Part model, mm, in its own coordinate system. Face numbers are marked on the shaded views. A direction names the side the tool comes from. Coordinates: 2 decimals unless noted, no trailing zeros. Write each loop counter-clockwise with the first axis right and the second up, starting at its lowest first coordinate (ties: lowest second). Pieces come first, ordered by that corner, then holes. Notation, with made-up numbers: (0.5, -21.75) -> (19.5, -21.75) arc R30 ccw to (19.5, 15.25) -> close; hole circle Ø2 at (29.25, 28.5). An arc over 180 degrees is marked (long way). Write item = value, one per line.
from build123d import *

# Parameters (mm, degrees)
F0_R     = 3.75
F0_R_2   = 2.5
F1_DEPTH = 15
F2_DEPTH = 9
F4_DEPTH = 7


# Not quite as in the source:
# - a feature names something its author has since deleted; it is built from what else it names


with BuildPart() as f1:
    # F0 (on Top) → F1 (new body)
    with BuildSketch(Plane.XY):
        Circle(F0_R)
        Circle(F0_R_2, mode=Mode.SUBTRACT)
    extrude(amount=F1_DEPTH)

    # F0 (on Top) → F2 (join)
    with BuildSketch(Plane.XY):
        Polygon((4.1, -2.3671361037), (4.1, 2.3671361037), (0, 4.7342722074), (-4.1, 2.3671361037), (-4.1, -2.3671361037), (0, -4.7342722074), align=None)
        Circle(F0_R, mode=Mode.SUBTRACT)
        Circle(F0_R)
        Circle(F0_R_2, mode=Mode.SUBTRACT)
        Circle(F0_R_2)
    extrude(amount=-F2_DEPTH)

    # F3 (on face) → F4 (cut)
    with BuildSketch(Plane(origin=(0, 0, -9), x_dir=(1, 0, 0), z_dir=(0, 0, -1))):
        Polygon((-3.3, 2.829016319), (-3.3, 0), (-3.3, -2.829016319), (-2.484232335, -3.3), (0, -3.3), (2.484232335, -3.3), (3.3, -2.829016319), (3.3, 0), (3.3, 2.829016319), (2.484232335, 3.3), (0, 3.3), (-2.484232335, 3.3), align=None)
    extrude(amount=-F4_DEPTH, mode=Mode.SUBTRACT)


solid = f1.part
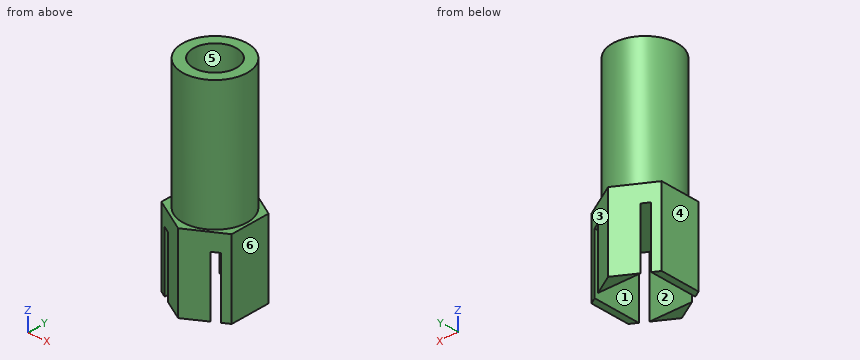
Q1. Which spindle directions (+Z, -Z, +X, -X, +Y, -Y) get a long thin tool onto all of the face, cutting with end or side? Do the marked faces 5 and 6. Say none if no direction does.
Model answer:
face_5 = +Z
face_6 = +Z, -Z, +X, +Y, -Y
Q2. Mould opens along X. For the marked faces 1, 2, 3 and 4 say: released by +X, released by -X, zero draft, split by the parting line, or undercut.
Model answer:
face_1 = undercut
face_2 = zero draft
face_3 = released by +X
face_4 = released by -X
Q3. Saw through at A-A on z = -6. Give the cut face in (x, y), and give its area (3 significant figures).
Model answer:
outline = (-4.1, -2.37) -> (-3.3, -2.83) -> (-3.3, 2.83) -> (-4.1, 2.37) -> close; (-2.48, -3.3) -> (0, -4.73) -> (2.48, -3.3) -> close; (-2.48, 3.3) -> (2.48, 3.3) -> (0, 4.73) -> close; (3.3, -2.83) -> (4.1, -2.37) -> (4.1, 2.37) -> (3.3, 2.83) -> close
area = 15.4 mm²
Q4. Saw through at D-D on z = -1. Give the cut face in (x, y), and give its area (3 significant figures).
Model answer:
outline = (-4.1, -2.37) -> (0, -4.73) -> (4.1, -2.37) -> (4.1, 2.37) -> (0, 4.73) -> (-4.1, 2.37) -> close
area = 58.2 mm²
Q5. Saw through at B-B on y = 0. Give the cut face in (x, z), and give its area (3 significant figures).
Model answer:
outline = (-4.1, -9) -> (-3.3, -9) -> (-3.3, -2) -> (3.3, -2) -> (3.3, -9) -> (4.1, -9) -> (4.1, 0) -> (3.75, 0) -> (3.75, 15) -> (2.5, 15) -> (2.5, 0) -> (-2.5, 0) -> (-2.5, 15) -> (-3.75, 15) -> (-3.75, 0) -> (-4.1, 0) -> close
area = 65.1 mm²
Q6. Pin check, flat tips, straight feed: pin 1 (2.5 mm diameter, centred on x = 0, y = 1, fed in from +Z); pin 2 (1.5 mm diameter, centred on x = -0.5, z = -5.5, fed in from +Y); pin 3 (1.5 mm diameter, centred on x = 1.5, z = 0, fed in from -Y). Stop position of each tip, or through.
Model answer:
pin_1 = 0
pin_2 = 4.73
pin_3 = -4.3
Q7. Probe line 1 (Y direction, x = 0, z = 7.25); line 2 (X direction, y = 0.5, z = -8); line 3 (Z direction, x = -1, y = -1.25). List the from-to ranges inside material, lowest first. Write a range as from..to.
Model answer:
line_1 = -3.75..-2.5, 2.5..3.75
line_2 = -4.1..-3.3, 3.3..4.1
line_3 = -2..0
Q8. Saw through at C-C on x = -1.75. Give the cut face in (y, z), and give its area (3 significant figures).
Model answer:
outline = (-3.72, -9) -> (-3.3, -9) -> (-3.3, -2) -> (3.3, -2) -> (3.3, -9) -> (3.72, -9) -> (3.72, 0) -> (3.32, 0) -> (3.32, 15) -> (1.79, 15) -> (1.79, 0) -> (-1.79, 0) -> (-1.79, 15) -> (-3.32, 15) -> (-3.32, 0) -> (-3.72, 0) -> close
area = 66.8 mm²
